Could you check a few things on this model? Use its own coordinates, in mm. A direction names the side the tool comes from. Round coordinates to 2 decimals unless told otherwise and drop trailing zeros. Loops run counter-clockwise (first coordinate to the right, second up) from the corner with the lowest first, then second, coordinate; pieces in that order, holes last. Notation, with made-up numbers: (26.5, 61) -> (57.5, 61) arc R34 ccw to (57.5, 98) -> close; hole circle Ø6 at (63.25, 20). An arc over 180 degrees is marked (long way). One line per item, written item: value.
Autodesk Inventor part; units mm, degrees
ref_plane "YZ Plane" through (0, 0, 0) normal (1, 0, 0) x (0, 1, 0)
ref_plane "XZ Plane" through (0, 0, 0) normal (0, 1, 0) x (-1, 0, 0)
ref_plane "XY Plane" through (0, 0, 0) normal (0, 0, 1) x (1, 0, 0)
sketch "Sketch1" plane through (0, 0, 0) normal (0, 1, 0) x (-1, 0, 0)
  line L0 (0, 0) -> (54, 0)
  line L1 (54, 0) -> (54, -10)
  line L2 (54, -10) -> (0, -10)
  line L3 (0, -10) -> (0, 0)
  line L4 (54, 0) -> (0, 0)
  line L5 (0, 0) -> (0, -2)
  line L6 (0, -2) -> (54, -2)
  line L7 (54, -2) -> (54, 0)
  dimension "d0" = 54
  dimension "d1" = 10
  dimension "d3" = 2
extrude "Extrusion1" add sketch "Sketch1" along normal blind 2 contours L6 L1 L2 L3
extrude "Extrusion2" add sketch "Sketch1" along normal blind 10 contours L0 L1 L6 L3
sketch "Sketch2" plane through (0, 0, -10) normal (1, 0, 0) x (0, 0, -1)
  line L0 (-10, 0) -> (0, 0)
  line L1 (-10, 0) -> (0, 0)
  line L2 (0, 0) -> (0, 10)
  line L3 (0, 10) -> (-10, 10)
  line L4 (-10, 10) -> (-10, 0)
  dimension "d8" = 10
  dimension "d9" = 10
extrude "Extrusion3" add sketch "Sketch2" against normal blind 2
sketch "Sketch3" plane through (-54, 0, -10) normal (-1, 0, 0) x (0, 0, 1)
  line L0 (0, 0) -> (0, 10)
  line L1 (10, 10) -> (0, 10)
  line L2 (0, 0) -> (10, 0)
  line L3 (10, 0) -> (10, 10)
  line L4 (10, 10) -> (0, 10)
  line L5 (0, 10) -> (0, 0)
  point P0 (10, 0)
extrude "Extrusion4" add sketch "Sketch3" against normal blind 2
sketch "Sketch5" plane through (0, 0, 0) normal (1, 0, 0) x (0, 0, -1)
  line L0 (10, 0) -> (10, 10)
  line L1 (0, 10) -> (10, 10)
  point P0 (0, 0)
  point P1 (6.5, 6.5)
  dimension "d19" = 3.5
  dimension "d20" = 3.5
hole "Hole1" at (0, 6.5, -6.5) direction (-1, 0, 0) diameter 4.5 depth 2
properties part number "Hinge Holder"
Item 1: If we section it at D-D on x = -29: List the corners of the cut face in (y, z) for me, plus the area to 3 significant figures.
Output:
outline: (0, -10) -> (2, -10) -> (2, -2) -> (10, -2) -> (10, 0) -> (0, 0) -> close
area: 36.0 mm²
Item 2: If we section it at B-B on y = 6.5: List the corners of the cut face in (x, z) for me, plus the area to 3 significant figures.
Output:
outline: (-54, -10) -> (-52, -10) -> (-52, -2) -> (-2, -2) -> (-2, -4.25) -> (0, -4.25) -> (0, 0) -> (-54, 0) -> close; (-2, -10) -> (0, -10) -> (0, -8.75) -> (-2, -8.75) -> close
area: 131 mm²
Item 3: If we section it at A-A on z = -6.5: List the corners of the cut face in (x, y) for me.
Output:
outline: (-54, 0) -> (0, 0) -> (0, 4.25) -> (-2, 4.25) -> (-2, 2) -> (-52, 2) -> (-52, 10) -> (-54, 10) -> close; (-2, 8.75) -> (0, 8.75) -> (0, 10) -> (-2, 10) -> close
Item 4: If we section it at C-C on z = -9.25: List the corners of the cut face in (x, y) for me, plus the area to 3 significant figures.
Output:
outline: (-54, 0) -> (0, 0) -> (0, 10) -> (-2, 10) -> (-2, 2) -> (-52, 2) -> (-52, 10) -> (-54, 10) -> close
area: 140 mm²
Item 5: I need wall thicknesses on line 1 (X direction, y = 2.5, z = -4.75); line 2 (Z direction, x = -0.4, y = 6.5); line 3 (Y direction, x = -1.1, z = -6.5). Which ranges of each line are inside material? Lowest first, please. Write a range as from..to.
Output:
line 1: x = -54..-52, -2..0
line 2: z = -10..-8.75, -4.25..0
line 3: y = 0..4.25, 8.75..10
Item 6: For faces 5 (the face through (-2, 6, -4)), 6 (the face through (-27, 1, -10)), which set-ups out of +Z, -Z, +X, -X, +Y, -Y let a thin tool reach every point of the face, with its end or its side?
Output:
face 5: -Z, +Y
face 6: -Z, +X, -X, +Y, -Y
Item 7: Will these pins go through, and if not, where does the flat tip stop? pin 1 Ø5 at (x, z) = (-24, -6) entering from +Y; pin 2 Ø4 at (y, z) = (4.5, -5) entering from +X; pin 3 Ø4 at (x, y) = (-36.5, 5.5) entering from -Z.
Output:
pin 1: stops at y = 2
pin 2: stops at x = 0
pin 3: stops at z = -2
Item 8: If we mould it in two halves opening along Y, with no side actions, what happens to faces 1 (the face through (-1.014, 5.824, -8.646)), 2 (the face through (-27, 0, -5)), 3 (the face through (-27, 6, -2)), 4 (the face through (-27, 2, -6))? For each: released by +Y, released by -Y, zero draft, split by the parting line, or undercut.
Output:
face 1: undercut
face 2: released by -Y
face 3: zero draft
face 4: released by +Y
